Work out the finished part from the listing and answer in its coordinate system (mm). Face numbers are marked on the shaded views. Give positions to 0.01 mm unless a question says otherwise; leave off trailing zeros. Loops run counter-clockwise (first coordinate to the right, second up) from the corner with the lowest first, then second, coordinate; pieces in that order, holes last. Notation, with made-up numbers: M -20.5,-23.5 L -10.5,-23.5 A7 cw -10.5,-19.5 Z; hole C 9.5,40.5 d5. An arc over 180 degrees is marked long. Use a Markdown table: item, result.
```python
from build123d import *

# Parameters (mm, degrees)
F1_ANGLE = 180


with BuildPart() as f1:
    # F0 (on Right) → F1 (revolve)
    with BuildSketch(Plane.YZ):
        with BuildLine():
            Line((-60.325, -6.35), (-60.325, 19.05))
            Line((-60.325, 19.05), (-63.5, 19.05))
            Line((-63.5, 19.05), (-63.5, -6.35))
            ThreePointArc((-63.5, -6.35), (-53.270704, -31.045704), (-28.575, -41.275))
            ThreePointArc((-28.575, -41.275), (-21.839808, -44.064808), (-19.05, -50.8))
            Line((-19.05, -50.8), (-19.05, -63.5))
            Line((-19.05, -63.5), (-15.875, -63.5))
            Line((-15.875, -63.5), (-15.875, -50.8))
            ThreePointArc((-15.875, -50.8), (-19.594744, -41.819744), (-28.575, -38.1))
            ThreePointArc((-28.575, -38.1), (-51.02564, -28.80064), (-60.325, -6.35))
        make_face()
    revolve(axis=Axis((0, 0, -17.790621), (0, 0, -1)), revolution_arc=F1_ANGLE)


solid = f1.part
```
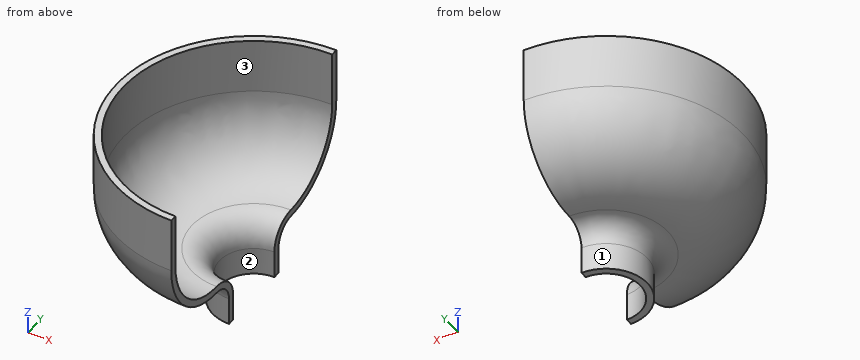
(1) Given P1, Ø8, axis at y = 42, z = -19.5, coming from the -X side; P2, Ø6, axis at y = -41, z = 8.5, coming from the +X side; P3, Ø6, axis at x = -46.5, y = -21.5, coming from the -Z side, each flat-ended and moving along its own axis, determine where each tip first touches the part or whether it passes through.
Entries:
| item | result |
|---|---|
| P1 | stops at x = -48.15 |
| P2 | stops at x = -41.27 |
| P3 | stops at z = -35.22 |
(2) The mould has two halves that part along Y. Classify the marked faces 1, 2 and 3: released by +Y, released by -Y, zero draft, split by the parting line, or undercut.
Entries:
| item | result |
|---|---|
| face 1 | split by the parting line |
| face 2 | undercut |
| face 3 | undercut |
(3) Consider probe 1 along Y at (x, z) = (-39, -24); probe 2 along Y at (x, z) = (-12, -15.5); probe 3 along X at (y, z) = (-48, -12.5). Determine where each line is inside the solid, lowest interval first. Write a range as [from, to].
Entries:
| item | result |
|---|---|
| probe 1 | y = [-43.89, -38.73], [38.73, 43.89] |
| probe 2 | y = [-61.11, -57.74], [57.74, 61.11] |
| probe 3 | x = [-40.73, -35.54] |
(4) A cutting plane is placed at A-A (z = -46). Write down the section's boundary in (x, y).
Entries:
| item | result |
|---|---|
| outline | M 0,-20.35 L 0,-16.82 A16.82 cw 0,16.82 L 0,20.35 A20.35 ccw Z |
